Part print with two shaded views. Sizes in mm from the minimum x, y, z corner. A direction names the side the tool comes from. Coordinates: 2 decimals unless noted, no trailing zeros. Write each loop counter-clockwise with the first axis right and the second up, starting at its lowest first coordinate (ties: lowest second). Pieces come first, ordered by that corner, then holes.
Q1. Band-saw the part on B-B, the plane y = 47. Write the cut outline in (x, z).
Q2. Band-saw the part on D-D, the plane y = 54.5. Write the cut outline in (x, z) (1 decimal).
Q3. Drill centre lines: probe 1 along X at (y, z) = (25, 45.5); probe 2 along Z at (x, y) = (5, 18.5); probe 3 along Y at (x, z) = (30.5, 4). Where is each one in solid material? Low to high.
Q4. Which spindle directions (+Z, -Z, +X, -X, +Y, -Y) get a long thin tool onto all of the face, cutting with end or side? Do the marked faces 4 and 5. Say none if no direction does.
Q5. Pull direction X, two halves, no side cores. Call the marked faces 1, 2 and 3: released by +X, released by -X, zero draft, split by the parting line, or undercut.
Q6. Pin check, flat tips, straight feed: P1, Ø4.5, axis at x = 17.1, y = 6.25, coming from the +Z side; P2, Ø1.6, axis at x = 43, y = 23, coming from the -Z side; P3, Ø1.6, axis at x = 1, z = 7.5, coming from the -Y side; P4, Ø2, axis at x = 10.5, z = 29.5, coming from the -Y side. Stop position of each tip, or through.
Q7. Band-saw the part on C-C, the plane z = 12. Write the cut outline in (x, y).
Q8. Band-saw the part on A-A, the plane x = 31. Write the cut outline in (y, z).
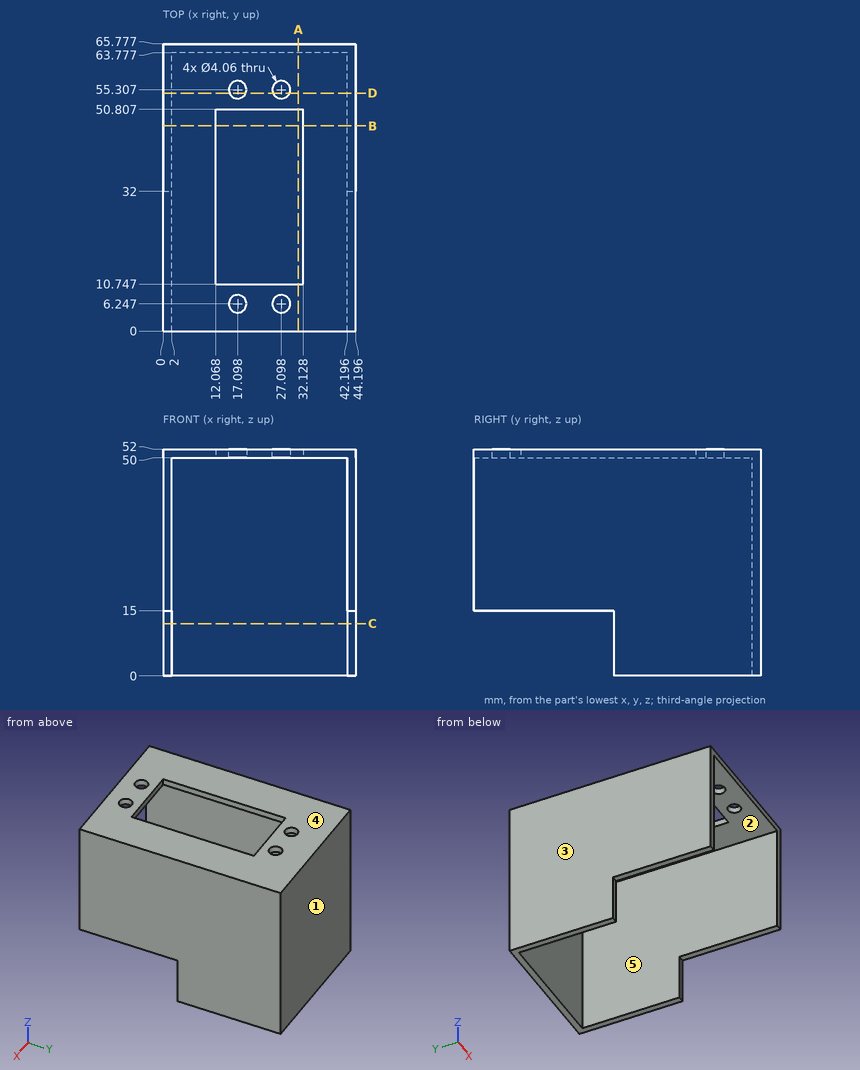
Answer sheet:
1. outline: (0, 0) - (2, 0) - (2, 50) - (12.07, 50) - (12.07, 52) - (0, 52) - close; (32.13, 50) - (42.2, 50) - (42.2, 0) - (44.2, 0) - (44.2, 52) - (32.13, 52) - close
2. outline: (0, 0) - (2, 0) - (2, 50) - (15.2, 50) - (15.2, 52) - (0, 52) - close; (19, 50) - (25.2, 50) - (25.2, 52) - (19, 52) - close; (29, 50) - (42.2, 50) - (42.2, 0) - (44.2, 0) - (44.2, 52) - (29, 52) - close
3. probe 1: x = 0 to 2, 42.2 to 44.2
3. probe 2: z = 50 to 52
3. probe 3: y = 63.78 to 65.78
4. face 4: +Z, +X, -X, +Y, -Y
4. face 5: -Z, -Y
5. face 1: zero draft
5. face 2: undercut
5. face 3: released by -X
6. P1: stops at z = 52
6. P2: stops at z = 15
6. P3: stops at y = 32
6. P4: stops at y = 63.78
7. outline: (0, 32) - (2, 32) - (2, 63.78) - (42.2, 63.78) - (42.2, 32) - (44.2, 32) - (44.2, 65.78) - (0, 65.78) - close
8. outline: (0, 50) - (10.75, 50) - (10.75, 52) - (0, 52) - close; (50.81, 50) - (63.78, 50) - (63.78, 0) - (65.78, 0) - (65.78, 52) - (50.81, 52) - close
